from build123d import *

# Parameters (mm, degrees)
SKETCH1_W           = 25
SKETCH1_H           = 14.7
BOSS_EXTRUDE1_DEPTH = 1
SKETCH2_W           = 5
SKETCH2_H           = 7.3
CUT_EXTRUDE1_DEPTH  = 1
SKETCH3_W           = 7.5
SKETCH3_H           = 5
CUT_EXTRUDE2_DEPTH  = 1
BOSS_EXTRUDE2_DEPTH = 1
SKETCH9_W           = 25
SKETCH9_H           = 14.7
BOSS_EXTRUDE3_DEPTH = 1
SKETCH11_W          = 22.5
SKETCH11_H          = 1
SKETCH11_W_2        = 2.5
SKETCH11_H_2        = 1.5
BOSS_EXTRUDE5_DEPTH = 1


with BuildPart() as part:
    # Sketch1 → Boss-Extrude1 (new body)
    with BuildSketch(Plane(origin=(0, 0, 0), x_dir=(1, 0, 0), z_dir=(0, 1, 0))):
        with Locations((-29.985488774, 13.606547542)):
            Rectangle(SKETCH1_W, SKETCH1_H)
    extrude(amount=BOSS_EXTRUDE1_DEPTH)

    # Sketch2 → Cut-Extrude1 (cut)
    with BuildSketch(Plane(origin=(0, 1, 0), x_dir=(1, 0, 0), z_dir=(0, 1, 0))):
        with Locations((-39.985488774, 14.606547542)):
            Rectangle(SKETCH2_W, SKETCH2_H)
    extrude(amount=-CUT_EXTRUDE1_DEPTH, mode=Mode.SUBTRACT)

    # Sketch3 → Cut-Extrude2 (cut)
    with BuildSketch(Plane(origin=(0, 1, 0), x_dir=(1, 0, 0), z_dir=(0, 1, 0))):
        with Locations((-21.235488774, 11.756547542)):
            Rectangle(SKETCH3_W, SKETCH3_H)
    extrude(amount=-CUT_EXTRUDE2_DEPTH, mode=Mode.SUBTRACT)

    # Sketch4 → Boss-Extrude2 (add)
    with BuildSketch(Plane.XZ):
        Polygon((-42.485488774, -6.256547542), (-42.485488774, -7.756547542), (-20.485488774, -7.756547542), (-20.485488774, -8.256547542), (-17.485488774, -8.256547542), (-17.485488774, -6.256547542), align=None)
        Polygon((-20.485488774, -19.456547542), (-42.485488774, -19.456547542), (-42.485488774, -20.956547542), (-17.485488774, -20.956547542), (-17.485488774, -18.456547542), (-20.485488774, -18.456547542), align=None)
    extrude(amount=BOSS_EXTRUDE2_DEPTH)

    # Sketch9 → Boss-Extrude3 (add)
    with BuildSketch(Plane(origin=(0, 1, 0), x_dir=(1, 0, 0), z_dir=(0, 1, 0))):
        with Locations((-29.985488774, 13.606547542)):
            Rectangle(SKETCH9_W, SKETCH9_H)
    extrude(amount=BOSS_EXTRUDE3_DEPTH)

    # Sketch11 → Boss-Extrude5 (add)
    with BuildSketch(Plane(origin=(0, -1, 0), x_dir=(-1, 0, 0), z_dir=(0, -1, 0))):
        with Locations((31.235488774, 6.756547542)):
            Rectangle(SKETCH11_W, SKETCH11_H)
        with Locations((18.735488774, 6.756547542)):
            Rectangle(SKETCH11_W_2, SKETCH11_H)
        with Locations((18.735488774, 7.756547542)):
            Rectangle(SKETCH11_W_2, SKETCH11_H)
        with Locations((18.735488774, 19.206547542)):
            Rectangle(SKETCH11_W_2, SKETCH11_H_2)
        with Locations((18.735488774, 20.456547542)):
            Rectangle(SKETCH11_W_2, SKETCH11_H)
        with Locations((31.235488774, 20.456547542)):
            Rectangle(SKETCH11_W, SKETCH11_H)
    extrude(amount=BOSS_EXTRUDE5_DEPTH)


solid = part.part
Read the model definition and answer for the solid it produces. Units are mm, in the model's axes. A direction names the side the tool comes from. Round coordinates to 2 decimals unless told otherwise and drop trailing zeros. Loops run counter-clockwise (first coordinate to the right, second up) from the corner with the lowest first, then second, coordinate; pieces in that order, holes last.
Q1. Which of the six approach directions +Z, -Z, +X, -X, +Y, -Y give full straight-line access (tool end or side, diameter ignored) to faces 4 (the face through (-24.985, 0.5, -11.7)), 5 (the face through (-17.485, 0.5, -15.3)), 6 (the face through (-19, -1, -8.257)), 7 (the face through (-30, 0, -20.957)), 8 (the face through (-31.1, -1.5, -19.957))?
Q2. Section D-D on z = -11.75 is taken. Write down the section's boundary in (x, y).
Q3. Section A-A on z = -19 is taken. Write down the section's boundary in (x, y), and give its area (3 significant figures).
Q4. Each of these flat-tipped pins is pushed along its axis until it touches: pin 1 (6 mm diameter, centred on x = -36, z = -14.5, fed in from -Y); pin 2 (0.5 mm diameter, centred on y = 0.5, z = -13, fed in from -X); pin 3 (0.8 mm diameter, centred on y = 0.5, z = -12, fed in from +X). Where does it stop, or does it pass through?
Q5. Section C-C on x = -29.25 is taken. Write down the section's boundary in (y, z), and give its area (3 significant figures).
Q6. Section B-B on y = -0.3 is taken. Write down the section's boundary in (x, z), and give its area (3 significant figures).
Q7. Determine the mould class of faces 1 (the face through (-30, -2, -7)), 2 (the face through (-31.4, -1, -7.5)), 3 (the face through (-30, 0, -6.257)) for opening direction Z: released by +Z, released by -Z, zero draft, split by the parting line, or undercut.
Q8. Consider probe 1 along Z at (x, y) = (-36.25, -0.35); probe 2 along Z at (x, y) = (-34.75, -1.15); probe 3 along Y at (x, z) = (-37.25, -18.25). Determine where each line is inside the solid, lowest interval first.
Output:
1. face 4: +X, -Y
1. face 5: +Z, -Z, +X, +Y, -Y
1. face 6: +X, -X, -Y
1. face 7: -Z, +X, -X, +Y, -Y
1. face 8: -X, -Y
2. outline: (-42.49, 1) - (-37.49, 1) - (-37.49, 0) - (-24.99, 0) - (-24.99, 1) - (-17.49, 1) - (-17.49, 2) - (-42.49, 2) - close
3. outline: (-42.49, 0) - (-20.49, 0) - (-20.49, -1) - (-19.99, -1) - (-19.99, -2) - (-17.49, -2) - (-17.49, 2) - (-42.49, 2) - close
3. area: 55.5 mm2
4. pin 1: stops at y = 0
4. pin 2: stops at x = -37.49
4. pin 3: stops at x = -24.99
5. outline: (-2, -20.96) - (2, -20.96) - (2, -6.26) - (-2, -6.26) - (-2, -7.26) - (-1, -7.26) - (-1, -7.76) - (0, -7.76) - (0, -19.46) - (-1, -19.46) - (-1, -19.96) - (-2, -19.96) - close
5. area: 34.4 mm2
6. outline: (-42.49, -20.96) - (-17.49, -20.96) - (-17.49, -18.46) - (-20.49, -18.46) - (-20.49, -19.46) - (-42.49, -19.46) - close; (-42.49, -7.76) - (-20.49, -7.76) - (-20.49, -8.26) - (-17.49, -8.26) - (-17.49, -6.26) - (-42.49, -6.26) - close
6. area: 79.5 mm2
7. face 1: zero draft
7. face 2: undercut
7. face 3: released by +Z
8. probe 1: z = -20.96 to -19.46, -7.76 to -6.26
8. probe 2: z = -20.96 to -19.96, -7.26 to -6.26
8. probe 3: y = 0 to 2
